Here's how the part is built. I have some questions about the finished solid (model axes, mm). Face numbers are marked on the shaded views. A direction names the side the tool comes from. Give positions to 0.01 mm unless a question says otherwise; leave off trailing zeros. Loops run counter-clockwise (first coordinate to the right, second up) from the corner with the lowest first, then second, coordinate; pieces in that order, holes last. Notation, with made-up numbers: (-40, 51.5) - (-9, 51.5) arc R26 cw to (-9, 71.5) - close; hole circle Ø3 at (33, 54). An arc over 180 degrees is marked (long way). Return JSON: item names as keys, results as strings. Group by question number.
(1) I need wall thicknesses on probe 1 along X at (y, z) = (37, -17.5); probe 2 along Y at (x, z) = (45, 0); probe 3 along Z at (x, y) = (47, 25). Which ranges of each line are inside material? Lowest first, please. Write a range as [from, to].
(2) On a 3-axis mill with a long thin cutter (end or side, diameter ignored), from which of +Z, -Z, +X, -X, +Y, -Y can I reach the whole of each face in a straight line? I mean the marked faces 1, 2 and 3. Say none if no direction works.
(3) If we section it at D-D (x = 0): Please give me the cut outline in (y, z), then the cut area to 3 significant figures.
(4) If we section it at B-B (y = 25.4): Please give me the cut outline in (x, z), then the cut area to 3 significant figures.
(5) If we section it at A-A (z = 0): Please give me the cut outline in (x, y).
(6) If we section it at C-C (y = 53): Please give me the cut outline in (x, z).
(7) If we mould it in two halves opening along X, with no side actions, what happens to the marked faces 4, 5, 6 and 7? For each: released by +X, released by -X, zero draft, split by the parting line, or undercut.
(8) For P1, Ø4, axis at x = 16, z = 7, coming from the -Y side; P2, Ø3, axis at x = 19.5, y = 124.5, coming from the +Z side; P3, Ø5, axis at y = 142, z = 12, coming from the +X side, each with a flat end and sliding along its axis, tell me the tip position at first contact or that it passes through.
```python
from build123d import *

# Parameters (mm, degrees)
SKETCH1_W           = 101.6
SKETCH1_H           = 76.2
BOSS_EXTRUDE1_DEPTH = 101.6
SKETCH2_W           = 76.2
SKETCH2_H           = 76.2
CUT_EXTRUDE1_DEPTH  = 63.5
SKETCH3_R           = 12.7
CUT_EXTRUDE2_DEPTH  = 149.649688866
SKETCH4_R           = 25.4
BOSS_EXTRUDE2_DEPTH = 76.2


with BuildPart() as part:
    # Sketch1 → Boss-Extrude1 (new body)
    with BuildSketch(Plane(origin=(0, 0, 0), x_dir=(1, 0, 0), z_dir=(0, 1, 0))):
        Rectangle(SKETCH1_W, SKETCH1_H)
    extrude(amount=BOSS_EXTRUDE1_DEPTH)

    # Sketch2 → Cut-Extrude1 (cut)
    with BuildSketch(Plane.XZ):
        Rectangle(SKETCH2_W, SKETCH2_H)
    extrude(amount=-CUT_EXTRUDE1_DEPTH, mode=Mode.SUBTRACT)

    # Sketch3 → Cut-Extrude2 (cut, through all)
    with BuildSketch(Plane(origin=(50.8, 0, 0), x_dir=(0, 0, -1), z_dir=(1, 0, 0))):
        with Locations((0, 25.4)):
            Circle(SKETCH3_R)
    extrude(amount=-CUT_EXTRUDE2_DEPTH, mode=Mode.SUBTRACT)

    # Sketch4 → Boss-Extrude2 (add)
    with BuildSketch(Plane(origin=(0, 101.6, 0), x_dir=(1, 0, 0), z_dir=(0, 1, 0))):
        with Locations(Location((0, 0, 0), (0, 0, 90))):
            Circle(SKETCH4_R)
    extrude(amount=BOSS_EXTRUDE2_DEPTH)


solid = part.part
```
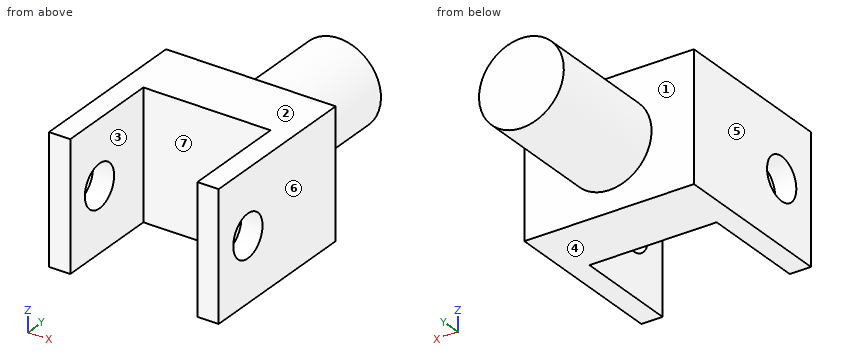
Values:
{
 "1": {"probe 1": "[-50.8, -38.1], [38.1, 50.8]", "probe 2": "[0, 12.7], [38.1, 101.6]", "probe 3": "[-38.1, -12.69], [12.69, 38.1]"},
 "2": {"face 1": "+Y", "face 2": "+Z, +X, -X, +Y, -Y", "face 3": "+Z, -Z, -Y"},
 "3": {"outline": "(63.5, -38.1) - (101.6, -38.1) - (101.6, -25.4) - (177.8, -25.4) - (177.8, 25.4) - (101.6, 25.4) - (101.6, 38.1) - (63.5, 38.1) - close", "area": "6,770 mm2"},
 "4": {"outline": "(-50.8, -38.1) - (-38.1, -38.1) - (-38.1, -12.7) - (-50.8, -12.7) - close; (-50.8, 12.7) - (-38.1, 12.7) - (-38.1, 38.1) - (-50.8, 38.1) - close; (38.1, -38.1) - (50.8, -38.1) - (50.8, -12.7) - (38.1, -12.7) - close; (38.1, 12.7) - (50.8, 12.7) - (50.8, 38.1) - (38.1, 38.1) - close", "area": "1,290 mm2"},
 "5": {"outline": "(-50.8, 0) - (-38.1, 0) - (-38.1, 12.7) - (-50.8, 12.7) - close; (-50.8, 38.1) - (-38.1, 38.1) - (-38.1, 63.5) - (38.1, 63.5) - (38.1, 38.1) - (50.8, 38.1) - (50.8, 101.6) - (25.4, 101.6) - (25.4, 177.8) - (-25.4, 177.8) - (-25.4, 101.6) - (-50.8, 101.6) - close; (38.1, 0) - (50.8, 0) - (50.8, 12.7) - (38.1, 12.7) - close"},
 "6": {"outline": "(-50.8, -38.1) - (-38.1, -38.1) - (-38.1, 38.1) - (-50.8, 38.1) - close; (38.1, -38.1) - (50.8, -38.1) - (50.8, 38.1) - (38.1, 38.1) - close"},
 "7": {"face 4": "zero draft", "face 5": "released by -X", "face 6": "released by +X", "face 7": "undercut"},
 "8": {"P1": "y = 63.5", "P2": "z = 17.92", "P3": "x = 23.56"}
}
